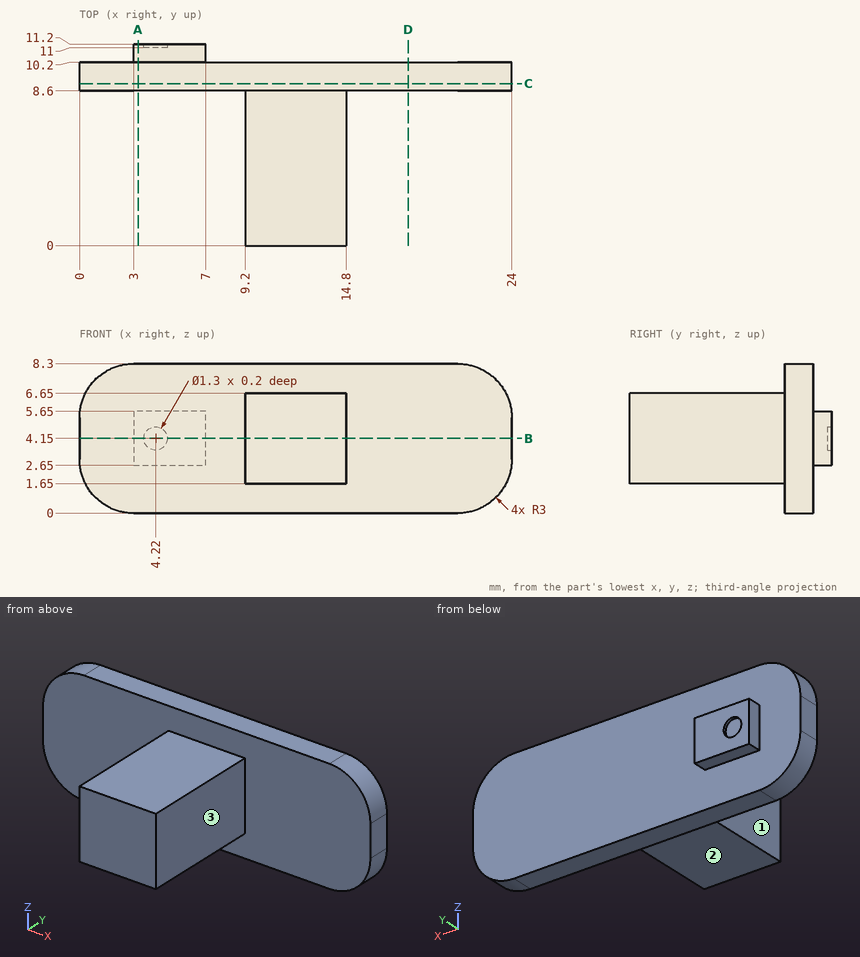
Drawing for the job (mm, zero at the part's lowest x, y, z). A direction names the side the tool comes from. Give positions to 0.01 mm unless a question says otherwise; leave off trailing zeros. Write each loop counter-clockwise with the first axis right and the second up, starting at its lowest first coordinate (ties: lowest second). Pieces come first, ordered by that corner, then holes. Notation, with made-up numbers: (63.5, -13.5) - (115.5, -13.5) arc R23 cw to (115.5, 2.5) - close; hole circle Ø3 at (32.25, 42). An arc over 180 degrees is marked (long way). Answer as CSV lines item,"result".
Q1. Drill centre lines: line 1 (Z direction, x = 4.22, y = 11.1); line 2 (X direction, y = 11.1, z = 4.15); line 3 (Z direction, x = 10.5, y = 7.5). Where is each one in solid material? Low to high. Write a range as from..to.
Result set:
line 1,"2.65..3.5, 4.8..5.65"
line 2,"3..3.57, 4.87..7"
line 3,"1.65..6.65"
Q2. Band-saw the part on D-D (x = 18.25). Give the cut face in (y, z).
Result set:
outline,"(8.6, 0) - (10.2, 0) - (10.2, 8.3) - (8.6, 8.3) - close"
Q3. Band-saw the part on A-A (x = 3.25). Give the cut face in (y, z), and give its area (3 significant figures).
Result set:
outline,"(8.6, 0) - (10.2, 0) - (10.2, 2.65) - (11.2, 2.65) - (11.2, 5.65) - (10.2, 5.65) - (10.2, 8.3) - (8.6, 8.3) - close"
area,"16.3 mm²"
Q4. 3-axis set-ups, long thin cutter, end or side, ignore diameter. For the marked faces 1, 2 and 3: which of +Z, -Z, +X, -X, +Y, -Y reach the whole face in a straight line?
Result set:
face 1,"+Z, -Z, -X, -Y"
face 2,"-Z, +X, -X, -Y"
face 3,"+Z, -Z, +X, -Y"
Q5. Band-saw the part on C-C (y = 9). Give the cut face in (x, z).
Result set:
outline,"(0, 3) arc R3 ccw to (3, 0) - (21, 0) arc R3 ccw to (24, 3) - (24, 5.3) arc R3 ccw to (21, 8.3) - (3, 8.3) arc R3 ccw to (0, 5.3) - close"
Q6. Flat gauge pins, fed straight in: pin 1 Ø1 at (x, z) = (20.5, 1) entering from -Y; pin 2 Ø4 at (y, z) = (5.5, 4.5) entering from +X; pin 3 Ø1.7 at (x, y) = (11.5, 2.5) entering from +Z. Where does each tip first touch, or does it go through?
Result set:
pin 1,"y = 8.6"
pin 2,"x = 14.8"
pin 3,"z = 6.65"
Q7. Band-saw the part on B-B (z = 4.15). Give the cut face in (x, y), and give its area (3 significant figures).
Result set:
outline,"(0, 8.6) - (9.2, 8.6) - (9.2, 0) - (14.8, 0) - (14.8, 8.6) - (24, 8.6) - (24, 10.2) - (7, 10.2) - (7, 11.2) - (4.87, 11.2) - (4.87, 11) - (3.57, 11) - (3.57, 11.2) - (3, 11.2) - (3, 10.2) - (0, 10.2) - close"
area,"90.3 mm²"
